For this review, take the finished solid that the model builds, in its own axes (mm). Face numbers are marked on the shaded views. A direction names the side the tool comes from. Coordinates: 2 decimals unless noted, no trailing zeros. Order: outer loops, then holes, each group sorted by start corner. A loop starts at its lowest first (then second) coordinate and runs counter-clockwise, first axis right, second up. Notation, with made-up numbers: (77, 67) - (83, 67) arc R15 ccw to (83, 91) - close; hole circle Ø3 at (83.25, 85.25). An arc over 180 degrees is marked (long way). One line per item, written item: value. Start each with the question number.
(1) Consider section A-A on y = 0. Write out the cut boundary in (x, z).
(2) Consider section B-B on x = 10.5. Write out the cut boundary in (y, z).
(3) Clearance check with flat-ended pins moving along their axes: pin 1 (10 mm diameter, centred on x = 41.5, y = 13.5, fed in from -Z); pin 2 (6 mm diameter, centred on x = 40, y = 27.5, fed in from +Z); pin 3 (17.5 mm diameter, centred on x = 28, y = 5, fed in from +Z). State where each tip first meets the part, or that it passes through.
(4) To check wall thickness, follow line 1 along Y through (x, z) = (34, 0); line 2 along Z through (x, y) = (25.5, 0.5); line 3 along X through (y, z) = (-38, -16). State the ranges of each line that lie inside material, in increasing order.
(5) Consider section D-D on z = -142.24. Write out the cut boundary in (x, y), then the cut area to 3 significant figures.
(6) Consider section C-C on z = 0. Write out the cut boundary in (x, y), then the cut area to 3 significant figures.
(7) For the marked faces 1 and 2, list the 3-axis set-ups (+Z, -Z, +X, -X, +Y, -Y) from which the entire face can be reached by the end or side of a thin tool; tool diameter is ignored.
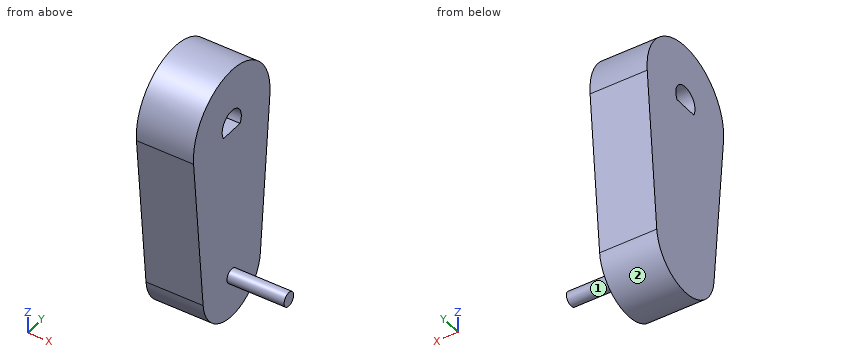
```python
from build123d import *

# Parameters (mm, degrees)
BOSS_EXTRUDE1_DEPTH = 50.8
SKETCH2_R           = 6.35
BOSS_EXTRUDE2_DEPTH = 50.8


with BuildPart() as part:
    # Sketch1 → Boss-Extrude1 (new body)
    with BuildSketch(Plane(origin=(0, 0, 0), x_dir=(0, 0, -1), z_dir=(1, 0, 0))):
        with BuildLine():
            Line((4.535714286, 50.597107585), (145.641785714, 37.947830688))
            ThreePointArc((145.641785714, 37.947830688), (180.34, 0), (145.641785714, -37.947830688))
            Line((145.641785714, -37.947830688), (4.535714286, -50.597107585))
            ThreePointArc((4.535714286, -50.597107585), (-50.8, 0), (4.535714286, 50.597107585))
        make_face()
        with BuildLine():
            Line((6.35, 10.998522628), (6.35, -10.998522628))
            ThreePointArc((6.35, -10.998522628), (-12.7, 0), (6.35, 10.998522628))
        make_face(mode=Mode.SUBTRACT)
    extrude(amount=BOSS_EXTRUDE1_DEPTH)

    # Sketch2 → Boss-Extrude2 (add)
    with BuildSketch(Plane(origin=(50.8, 0, 0), x_dir=(0, 0, -1), z_dir=(1, 0, 0))):
        with Locations((142.24, 0)):
            Circle(SKETCH2_R)
    extrude(amount=BOSS_EXTRUDE2_DEPTH)


solid = part.part
```
Geometry check:
1. outline: (0, -180.34) - (50.8, -180.34) - (50.8, -148.59) - (101.6, -148.59) - (101.6, -135.89) - (50.8, -135.89) - (50.8, -6.35) - (0, -6.35) - close; (0, 12.7) - (50.8, 12.7) - (50.8, 50.8) - (0, 50.8) - close
2. outline: (-50.6, -4.54) - (-37.95, -145.64) arc R38.1 ccw to (37.95, -145.64) - (50.6, -4.54) arc R50.8 ccw (long way) to start; hole (-11, -6.35) - (11, -6.35) arc R12.7 ccw (long way) to start
3. pin 1: stops at z = -179.38
3. pin 2: stops at z = 44.5
3. pin 3: stops at z = 50.8
4. line 1: y = -50.8 to -12.7, 12.7 to 50.8
4. line 2: z = -180.34 to -6.35, 12.69 to 50.8
4. line 3: x = 0 to 50.8
5. outline: (0, -38.25) - (50.8, -38.25) - (50.8, -6.35) - (101.6, -6.35) - (101.6, 6.35) - (50.8, 6.35) - (50.8, 38.25) - (0, 38.25) - close
5. area: 4,530 mm^2
6. outline: (0, -50.8) - (50.8, -50.8) - (50.8, -12.7) - (0, -12.7) - close; (0, 12.7) - (50.8, 12.7) - (50.8, 50.8) - (0, 50.8) - close
6. area: 3,870 mm^2
7. face 1: +X
7. face 2: -Z, +X, -X
